```python
from build123d import *

# Parameters (mm, degrees)
F0_W      = 3
F0_H      = 1.5
F0_W_2    = 2
F0_H_2    = 3.5
F0_W_3    = 1
F0_W_4    = 8
F1_DEPTH  = 9
F5_DEPTH  = 25
F7_DEPTH  = 25
F9_DEPTH  = 25
F10_W     = 3
F10_H     = 0.6
F11_DEPTH = 25
F12_SIZE2 = 1.75
F12_SIZE  = 1.75
F13_SIZE2 = 1.74999
F13_SIZE  = 1.74999


# Not quite as in the source:
# - a fillet or chamfer is up to 0.001 mm smaller than in the source, because OpenCascade refuses the exact size


with BuildPart() as f1:
    # F0 (on Top) → F1 (new body)
    with BuildSketch(Plane.XY):
        Polygon((4.1984589845, 2.5), (-9.8015410155, 2.5), (-9.8015410155, 0.75), (-9.8015410155, -0.75), (-9.8015410155, -2.5), (4.1984589845, -2.5), (4.1984589845, -1.75), (15.1984589845, -1.75), (15.1984589845, 1.75), (4.1984589845, 1.75), align=None)
        with Locations((-11.3015410155, 0)):
            Rectangle(F0_W, F0_H)
        with Locations((16.1984589845, 0)):
            Rectangle(F0_W_2, F0_H_2)
        with Locations((17.6984589845, 0)):
            Rectangle(F0_W_3, F0_H_2)
        with Locations((22.1984589845, 0)):
            Rectangle(F0_W_4, F0_H_2)
    extrude(amount=-F1_DEPTH)

    # F4 (on offset) → F5 (cut)
    with BuildSketch(Plane(origin=(0, 2.5, 0), x_dir=(-1, 0, 0), z_dir=(0, 1, 0))):
        Polygon((-26.1984589845, -7), (-24.1984589845, -5), (-23.1984589845, -5), (-23.1984589845, -1.5), (-22.1984589845, 0), (-26.1984589845, 0), align=None)
        Polygon((-18.1984589845, 0), (-20.1984589845, 0), (-19.1984589845, -1.5), (-18.1984589845, -1.5), align=None)
    extrude(amount=-F5_DEPTH, mode=Mode.SUBTRACT)

    # F6 (on face) → F7 (cut)
    with BuildSketch(Plane.XZ.offset(1.75)):
        Polygon((4.1984589845, -9), (18.1984589845, -9), (18.1984589845, -7), (17.1984589845, -7), (15.1984589845, -5), (4.1984589845, -5), align=None)
        Polygon((8.6984589845, -0.75), (9.1984589845, 0), (4.1984589845, 0), (4.1984589845, -1.5), (5.6984589845, -1.5), (6.6984589845, -0.75), align=None)
        Polygon((15.1984589845, -1.5), (18.1984589845, -1.5), (18.1984589845, 0), (13.1984589845, 0), (14.1984589845, -1.5), align=None)
    extrude(amount=-F7_DEPTH, mode=Mode.SUBTRACT)

    # F8 (on face) → F9 (cut)
    with BuildSketch(Plane.XZ.offset(2.5)):
        Polygon((-12.8015410155, -9), (4.1984589845, -9), (4.1984589845, -5), (-10.3015410155, -5), (-12.8015410155, -5), align=None)
        Polygon((4.1984589845, -1.5), (4.1984589845, 0), (-12.8015410155, 0), (-12.8015410155, -3.1837357674), (-10.3015410155, -3.1837357674), (-10.3015410155, -3.4337357674), (-8.3015410155, -3.4337357674), (-8.3015410155, -1.5), align=None)
    extrude(amount=-F9_DEPTH, mode=Mode.SUBTRACT)

    # F10 (on face) → F11 (cut)
    with BuildSketch(Plane.XZ.offset(2.5)):
        Polygon((-9.8015410155, -5), (-6.6717453301, -5), (-6.6717453301, -4.5), (6.6984589845, -4.5), (6.6984589845, -3.8), (-9.8015410155, -3.8), (-9.8015410155, -4.4), align=None)
        with Locations((-11.3015410155, -4.7)):
            Rectangle(F10_W, F10_H)
    extrude(amount=-F11_DEPTH, mode=Mode.SUBTRACT)

    # F12
    f12_edges = [f1.edges().sort_by_distance(p)[0] for p in [
        (21.198459, -1.75, 0),
    ]]
    chamfer(f12_edges, length=F12_SIZE, length2=F12_SIZE2)

    # F13 (size 1.75 and 1.75 in the source; OpenCascade refuses exactly that, so slightly less here)
    f13_edges = [f1.edges().sort_by_distance(p)[0] for p in [
        (21.198459, 1.75, 0),
    ]]
    chamfer(f13_edges, length=F13_SIZE, length2=F13_SIZE2)


solid = f1.part
```
For this review, take the finished solid that the model builds, in its own axes (mm). A direction names the side the tool comes from. Give positions to 0.01 mm unless a question says otherwise; leave off trailing zeros. Order: outer loops, then holes, each group sorted by start corner. A loop starts at its lowest first (then second) coordinate and runs counter-clockwise, first axis right, second up.
1) Insertion check: pin 1 (0.6 mm diameter, centred on x = -11.5, z = -4, fed in from -Y); pin 2 (1.5 mm diameter, centred on y = -1.5, z = -5, fed in from -X); pin 3 (0.6 mm diameter, centred on y = -2, z = -4.5, fed in from +X). Each pin has a flat end and moves straight along its axis. Give the tip position at first contact, or say it passes through.
2) Wall thickness on line 1 (Z direction, x = 5, y = 0.5); line 2 (X direction, y = 0.1, z = -8); line 3 (X direction, y = 1.8, z = -3): over which ranges is each line inside the solid? List them lowest first.
3) Take a section at A-A (x = -2). Give the boundary of the cut face in (y, z), then the cut area to 3 significant figures.
4) The part is to be moulded in two halves that separate along X. For faces 4 (the face through (17, -1.75, -5)), 5 (the face through (-1, 0, -3.8)), 6 (the face through (-9, 0, -3.434)), 7 (the face through (-12.802, 0, -4)), say which applies: released by +X, released by -X, zero draft, split by the parting line, or undercut.
5) Take a section at C-C (z = -7.75). Give the boundary of the cut face in (x, y), then the cut area to 3 significant figures.
6) For faces 1 (the face through (-1, 0, -1.5)), 2 (the face through (-11, 0.75, -4)), 3 (the face through (18.198, 0, -8)), list the 3-axis set-ups (+Z, -Z, +X, -X, +Y, -Y) from which the entire face can be reached by the end or side of a thin tool; tool diameter is ignored.
Derived:
1. pin 1: stops at y = -0.75
1. pin 2: stops at x = -6.67
1. pin 3: stops at x = 23.2
2. line 1: z = -5 to -4.5, -3.8 to -1.5
2. line 2: x = 18.2 to 26.2
2. line 3: x = -8.3 to 4.2
3. outline: (-2.5, -5) - (2.5, -5) - (2.5, -4.5) - (-2.5, -4.5) - close; (-2.5, -3.8) - (2.5, -3.8) - (2.5, -1.5) - (-2.5, -1.5) - close
3. area: 14.0 mm2
4. face 4: zero draft
4. face 5: undercut
4. face 6: undercut
4. face 7: released by -X
5. outline: (18.2, -1.75) - (26.2, -1.75) - (26.2, 1.75) - (18.2, 1.75) - close
5. area: 28.0 mm2
6. face 1: +Z, -X, +Y, -Y
6. face 2: +Z, -Z, -X, +Y
6. face 3: -Z, -X, +Y, -Y
